Input: dimensioned drawing with shaded views. Units: mm. Origin: part minimum x, y, z. A direction names the side the tool comes from. Give positions to 0.01 mm unless a question says otherwise; leave off trailing zeros. Order: outer loops, then holes, each group sorted by start corner. A loop starts at its lowest first (then second) coordinate and runs counter-clockwise, first axis right, second up.
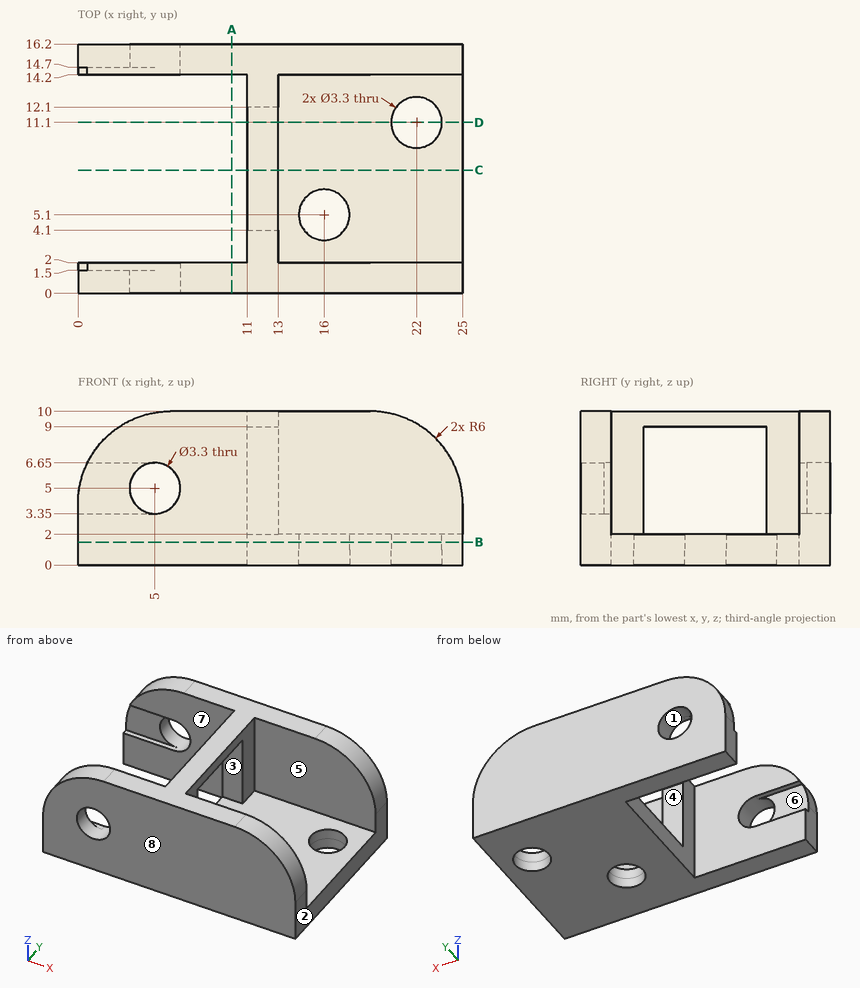
1) Draft query along X for the marked faces 1, 2 and 3. Return one class per face: +X half, -X half, draft (parallel to the pull), parting line (faces both ways), or undercut.
Report:
face 1: undercut
face 2: +X half
face 3: draft
2) Section query A-A, the plane x = 10. Return the cut outline in (y, z), and give its area (3 significant figures).
Report:
outline: (0, 0) - (2, 0) - (2, 10) - (0, 10) - close; (14.2, 0) - (16.2, 0) - (16.2, 10) - (14.2, 10) - close
area: 40.0 mm2
3) Section query C-C, the plane y = 8. Return the cut outline in (x, z).
Report:
outline: (11, 0) - (25, 0) - (25, 2) - (11, 2) - close; (11, 9) - (13, 9) - (13, 10) - (11, 10) - close
4) Pin query (flat end, axial travel): pin 1 (6 mm diameter, centred on y = 6.5, z = 7, fed in from +X); pin 2 (0.6 mm diameter, centred on x = 2, y = 14.5, fed in from +Z); pin 3 (4.5 mm diameter, centred on x = 22, y = 11.1, fed in from +Z). Return the tip coordinate at first contact, or that it passes through.
Report:
pin 1: stops at x = 13
pin 2: stops at z = 8.72
pin 3: stops at z = 2
5) Material intervals for L1, parallel to Y at x = 20.75, z = 6.5; L2, parallel to Y at x = 22, z = 1.65; L3, parallel to X at y = 12.25, z = 4.25, sorted ascending.
Report:
L1: y = 0 to 2, 14.2 to 16.2
L2: y = 0 to 9.45, 12.75 to 16.2
L3: x = 11 to 13
6) Section query B-B, the plane z = 1.5. Return the cut outline in (x, y).
Report:
outline: (0, 0) - (25, 0) - (25, 16.2) - (0, 16.2) - (0, 14.2) - (11, 14.2) - (11, 2) - (0, 2) - close; hole circle Ø3.3 at (16, 5.1); hole circle Ø3.3 at (22, 11.1)
7) Reachability of the marked faces 4, 5, 6, 7 and 8 from +Z, -Z, +X, -X, +Y, -Y: full face, straight path, thin tool, end or side. Return the list, or none.
Report:
face 4: +X, -X
face 5: +Z, +X
face 6: -X
face 7: +Z, -Z, -X
face 8: +Z, -Z, +X, -X, -Y
8) Section query D-D, the plane y = 11.1. Return the cut outline in (x, z).
Report:
outline: (11, 0) - (20.35, 0) - (20.35, 2) - (11, 2) - close; (11, 9) - (13, 9) - (13, 10) - (11, 10) - close; (23.65, 0) - (25, 0) - (25, 2) - (23.65, 2) - close
